Design review of the part built by this model. Coordinates are the model's own, in mm. A direction names the side the tool comes from. Round coordinates to 2 decimals unless told otherwise and drop trailing zeros. Order: outer loops, then holes, each group sorted by start corner. A loop starts at its lowest first (then second) coordinate and runs counter-clockwise, first axis right, second up. Notation, with made-up numbers: M -3.75,-37 L 22.25,-37 A10 ccw 22.25,-31 Z; hole C 7,74 d8. An arc over 180 degrees is marked long. Write item = value, one per line. Start each with the question number.
```python
from build123d import *

# Parameters (mm, degrees)
CROQUIS1_R              = 3.556
SALIENTE_EXTRUIR1_DEPTH = 3.1242
SALIENTE_EXTRUIR3_START = -3.1242
SALIENTE_EXTRUIR3_DEPTH = 3.1242
CROQUIS3_R              = 1.016
CORTAR_EXTRUIR1_DEPTH   = 45.69699718


with BuildPart() as part:
    # Croquis1 → Saliente-Extruir1 (new body)
    with BuildSketch(Plane.XY):
        with BuildLine():
            Line((9.525, 0), (9.525, 33.3375))
            ThreePointArc((9.525, 33.3375), (0, 42.8625), (-9.525, 33.3375))
            Line((-9.525, 33.3375), (-9.525, 0))
            ThreePointArc((-9.525, 0), (0, -9.525), (9.525, 0))
        make_face()
        Circle(CROQUIS1_R, mode=Mode.SUBTRACT)
        with BuildLine():
            ThreePointArc((-5.9055, 26.9875), (0, 21.082), (5.9055, 26.9875))
            Line((5.9055, 26.9875), (5.9055, 33.3375))
            ThreePointArc((5.9055, 33.3375), (0, 39.243), (-5.9055, 33.3375))
            Line((-5.9055, 33.3375), (-5.9055, 26.9875))
        make_face(mode=Mode.SUBTRACT)
        with BuildLine():
            ThreePointArc((1.524, 12.7), (0, 14.224), (-1.524, 12.7))
            Line((-1.524, 12.7), (-1.524, 6.35))
            ThreePointArc((-1.524, 6.35), (0, 4.826), (1.524, 6.35))
            Line((1.524, 6.35), (1.524, 12.7))
        make_face(mode=Mode.SUBTRACT)
    extrude(amount=SALIENTE_EXTRUIR1_DEPTH)

    # Croquis2 → Saliente-Extruir3 (add)
    with BuildSketch(Plane.XY.offset(3.1242).offset(SALIENTE_EXTRUIR3_START)):
        with BuildLine():
            ThreePointArc((-9.525, 33.3375), (-6.735192091, 40.072692091), (0, 42.8625))
            ThreePointArc((0, 42.8625), (-9.233702216, 38.679444926), (-12.178104888, 28.979460428))
            ThreePointArc((-12.178104888, 28.979460428), (-11.736773179, 27.137352023), (-10.922866894, 25.426886118))
            ThreePointArc((-10.922866894, 25.426886118), (-9.881124174, 23.039641343), (-9.525, 20.459458969))
            Line((-9.525, 20.459458969), (-9.525, 29.1465))
            ThreePointArc((-9.525, 29.1465), (-10.541, 30.1625), (-9.525, 31.1785))
            Line((-9.525, 31.1785), (-9.525, 33.3375))
        make_face()
        with BuildLine():
            ThreePointArc((12.178104888, 28.979460428), (9.233702216, 38.679444926), (0, 42.8625))
            ThreePointArc((0, 42.8625), (6.735192091, 40.072692091), (9.525, 33.3375))
            Line((9.525, 33.3375), (9.525, 31.1785))
            ThreePointArc((9.525, 31.1785), (10.541, 30.1625), (9.525, 29.1465))
            Line((9.525, 29.1465), (9.525, 20.459458969))
            ThreePointArc((9.525, 20.459458969), (9.881124174, 23.039641343), (10.922866894, 25.426886118))
            ThreePointArc((10.922866894, 25.426886118), (11.736773179, 27.137352023), (12.178104888, 28.979460428))
        make_face()
    extrude(amount=SALIENTE_EXTRUIR3_DEPTH)

    # Croquis3 → Cortar-Extruir1 (cut, through all)
    with BuildSketch(Plane.XY.offset(3.1242)):
        with Locations((-9.525, 30.1625)):
            Circle(CROQUIS3_R)
        with Locations((9.525, 30.1625)):
            Circle(CROQUIS3_R)
    extrude(amount=-CORTAR_EXTRUIR1_DEPTH, mode=Mode.SUBTRACT)


solid = part.part
```
(1) Consider section D-D, the plane x = -8. Write out the cut boundary in (y, z), then the cut area to 3 significant figures.
(2) Consider section C-C, the plane y = 23. Write out the cut boundary in (x, z).
(3) Insertion check: pin 1 (1.6 mm diameter, centred on y = 8.5, z = 1.5, fed in from +X) (3 decimals); pin 2 (0.9 mm diameter, centred on y = 8.5, z = 1, fed in from -X) (3 decimals); pin 3 (1.5 mm diameter, centred on x = -2, z = 0.5, fed in from -Y). Each pin has a flat end and moves straight along its axis. Give the tip position at first contact, or say it passes through.
(4) For faces 5 (the face through (9.525, 10, 2)), 6 (the face through (0, 17, 0)), 7 (the face through (-9.525, 10, 2)), 8 (the face through (-0.209, -9.523, 1.54)), 9 (the face through (-0.034, 4.826, 1.54)), list the 3-axis set-ups (+Z, -Z, +X, -X, +Y, -Y) from which the entire face can be reached by the end or side of a thin tool; tool diameter is ignored.
(5) Consider section B-B, the plane z = 0.5. State how many separate pieces and enclosed holes the cut face has, then the cut area to 3 significant figures.
(6) Draft analysis for pull direction X (two halves, no side actions). For faces 1 (the face through (-0.13, 21.083, 1.54)), 2 (the face through (1.524, 9, 2)), 3 (the face through (-9.9, 23.1, 1.5)), 4 (the face through (9.87, 23, 1.54)), state which applies: pulls with the +X half, pulls with the -X half, needs draft (parallel to the pull), parting line crosses it, or undercut.
(7) For line 1 along Y through (x, z) = (0, 1.5) (1 decimal); line 2 along X through (y, z) = (8, 2.7) (3 decimals); line 3 along X through (y, z) = (4.5, 1.4) (3 decimals), list the stretches that pass through material, from the lowest coordinate up. Write a range as [from, to].
(8) Consider section A-A, the plane y = 8.5. Write out the cut boundary in (x, z) (3 decimals).
Completed:
q1.outline = M -5.17,0 L 39.9,0 L 39.9,3.12 L -5.17,3.12 Z
q1.area = 141 mm2
q2.outline = M -9.87,0 L -4.36,0 L -4.36,3.12 L -9.87,3.12 Z; M 4.36,0 L 9.87,0 L 9.87,3.12 L 4.36,3.12 Z
q3.pin_1 = 9.525
q3.pin_2 = -9.525
q3.pin_3 = -9.44
q4.face_5 = +Z, -Z, +X, -Y
q4.face_6 = -Z, +X, -X, +Y, -Y
q4.face_7 = +Z, -Z, -X, -Y
q4.face_8 = +Z, -Z, -Y
q4.face_9 = +Z, -Z
q5.separate_pieces = 1
q5.enclosed_holes = 5
q5.area = 733 mm2
q6.face_1 = undercut
q6.face_2 = undercut
q6.face_3 = pulls with the -X half
q6.face_4 = pulls with the +X half
q7.line_1 = [-9.5, -3.6], [3.6, 4.8], [14.2, 21.1], [39.2, 42.9]
q7.line_2 = [-9.525, -1.524], [1.524, 9.525]
q7.line_3 = [-9.525, 9.525]
q8.outline = M -9.525,0 L -1.524,0 L -1.524,3.124 L -9.525,3.124 Z; M 1.524,0 L 9.525,0 L 9.525,3.124 L 1.524,3.124 Z
